Geometry: final body of the model. Coordinates: model frame, mm. Face numbers are marked on the shaded views. Give positions to 0.01 mm unless a question says otherwise; leave off trailing zeros. Write each loop counter-clockwise with the first axis right and the second up, starting at its lowest first coordinate (ties: lowest second). Pieces come first, ordered by that corner, then holes. Notation, with made-up numbers: M -23.75,53 L -1.75,53 A17 ccw -1.75,61 Z; hole C -6.75,43.5 d8. An arc over 180 degrees is marked long. Use a Markdown table: item, result. Add a question column.
(1) Draft query along Z for the marked faces 1, 2 and 3. Return one class per face: released by +Z, released by -Z, zero draft, split by the parting line, or undercut.
(2) Cut plane D-D (y = -31.5). Output: boundary loops of the cut face in (x, z).
(3) Material intervals for L1, parallel to Y at x = 10, z = 2.7; L2, parallel to Z at x = 22, y = -14; L3, parallel to Y at x = 21, z = -36, sorted ascending.
(4) Cut plane B-B (y = -45.5). Output: boundary loops of the cut face in (x, z), plus the area to 3 significant figures.
(5) Pin query (flat end, axial travel): pin 1 Ø6 at (x, z) = (18, -30.5) entering from +Y; pin 2 Ø5 at (y, z) = (-45.5, -5.5) entering from -X; pin 3 Ø1.2 at (x, z) = (56.5, 1.5) entering from -Y. Return the tip coordinate at first contact, or that it passes through.
(6) Cut plane C-C (z = -21). Output: boundary loops of the cut face in (x, y).
(7) Cut plane A-A (z = -36.5). Output: boundary loops of the cut face in (x, y), plus the area to 3 significant figures.
```python
from build123d import *
from OCP.BRepFilletAPI import BRepFilletAPI_MakeChamfer

# Parameters (mm, degrees)
BOSS_EXTRU_1_DEPTH   = 4
ESQUISSE3_R          = 12.5
BOSS_EXTRU_2_DEPTH   = 6
D_GAGEMENT_M31_D     = 3.2
D_GAGEMENT_M41_D     = 4.3
D_GAGEMENT_M41_DEPTH = 15
CONG_1_R             = 2
CHANFREIN1_SIZE      = 4
CHANFREIN1_SIZE2     = 15.704369422
CONG_2_R             = 10


with BuildPart() as part:
    # Esquisse1 → Boss.-Extru.1 (new body)
    with BuildSketch(Plane.XY):
        Polygon((0, 0), (0, -80), (25, -80), (25, -20), (83, -20), (83, 0), align=None)
    extrude(amount=BOSS_EXTRU_1_DEPTH)

    # Esquisse3 → Boss.-Extru.2 (add)
    with BuildSketch(Plane(origin=(25, 0, 0), x_dir=(0, 0, -1), z_dir=(1, 0, 0))):
        Polygon((0, -9), (42, -9), (42, -51), (0, -80), align=None)
        with Locations((21, -30)):
            Circle(ESQUISSE3_R, mode=Mode.SUBTRACT)
    extrude(amount=-BOSS_EXTRU_2_DEPTH)

    # Dégagement M31 (through all)
    with Locations(Plane(origin=(25, 0, 0), x_dir=(0, 0, -1), z_dir=(1, 0, 0))):
        with Locations((5.5, -14.5), (36.5, -14.5), (36.5, -45.5), (5.5, -45.5)):
            Hole(D_GAGEMENT_M31_D / 2)

    # Dégagement M41
    with Locations(Plane.XY.offset(4)):
        with Locations((10, -10), (10, -70), (77, -10)):
            Hole(D_GAGEMENT_M41_D / 2, depth=D_GAGEMENT_M41_DEPTH)

    # Congé1
    cong_1_edges = [part.edges().sort_by_distance(p)[0] for p in [
        (19, -44.5, 0),
        (22, -9, 0),
    ]]
    fillet(cong_1_edges, radius=CONG_1_R)

    # Chanfrein1: one chamfer whose edges measure the first distance from different faces: ONE call of the kernel's chamfer builder (chamfer() names one face for all edges)
    chanfrein1_edges_1 = [part.edges().sort_by_distance(p)[0] for p in [
        (22, -9, -42),
    ]]
    chanfrein1_edges_2 = [part.edges().sort_by_distance(p)[0] for p in [
        (22, -51, -42),
    ]]
    chanfrein1_side_2 = [part.faces().sort_by_distance(p)[0] for p in [
        (22, -30, -42),
    ]]
    chanfrein1 = BRepFilletAPI_MakeChamfer(part.part.solid().wrapped)
    for e in chanfrein1_edges_1:
        chanfrein1.Add(CHANFREIN1_SIZE, e.wrapped)
    for e in chanfrein1_edges_2:
        chanfrein1.Add(CHANFREIN1_SIZE, CHANFREIN1_SIZE2, e.wrapped, chanfrein1_side_2[0].wrapped)  # the first distance lies on this face
    add(Compound.cast(chanfrein1.Shape()), mode=Mode.REPLACE)

    # Congé2
    cong_2_edges = [part.edges().sort_by_distance(p)[0] for p in [
        (83, -20, 2),
        (0, -80, 2),
        (0, 0, 2),
        (83, 0, 2),
    ]]
    fillet(cong_2_edges, radius=CONG_2_R - 0.0001)  # a hair under: the kernel refuses the full size


solid = part.part
```
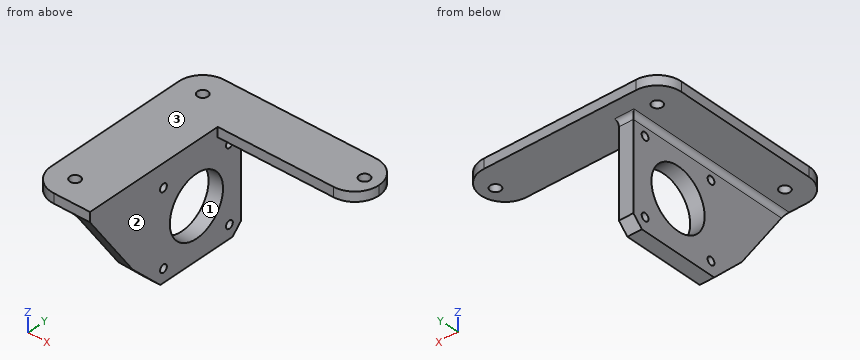
Answer list:
| question | item | result |
|---|---|---|
| 1 | face 1 | undercut |
| 1 | face 2 | zero draft |
| 1 | face 3 | released by +Z |
| 2 | outline | M 0,0 L 17,0 A2 cw 19,-2 L 19,-8.59 L 25,-8.59 L 25,4 L 0,4 Z; M 19,-42 L 25,-42 L 25,-33.41 L 19,-33.41 Z |
| 3 | L1 | -80 to -72.15, -67.85 to -12.15, -7.85 to 0 |
| 3 | L2 | -42 to -38.02, -34.98 to -7.02, -3.98 to 4 |
| 3 | L3 | -53 to -47.02, -43.98 to -16.02, -12.98 to -9 |
| 4 | outline | M 0,0 L 17,0 A2 cw 19,-2 L 19,-3.9 L 25,-3.9 L 25,4 L 0,4 Z; M 19,-42 L 25,-42 L 25,-38.1 L 19,-38.1 Z; M 19,-34.9 L 25,-34.9 L 25,-7.1 L 19,-7.1 Z |
| 4 | area | 314 mm² |
| 5 | pin 1 | y = -9 |
| 5 | pin 2 | x = 19 |
| 5 | pin 3 | y = -20 |
| 6 | outline | M 19,-65.5 L 25,-65.5 L 25,-42.5 L 19,-42.5 Z; M 19,-17.5 L 25,-17.5 L 25,-9 L 19,-9 Z |
| 7 | outline | M 19,-52.5 L 25,-52.5 L 25,-47.1 L 19,-47.1 Z; M 19,-43.9 L 25,-43.9 L 25,-16.1 L 19,-16.1 Z; M 19,-12.9 L 25,-12.9 L 25,-9 L 19,-9 Z |
| 7 | area | 223 mm² |
